Here's how the part is built. I have some questions about the finished solid (model axes, mm). Face numbers are marked on the shaded views. Coordinates: 2 decimals unless noted, no trailing zeros. Loops run counter-clockwise (first coordinate to the right, second up) from the corner with the lowest first, then second, coordinate; pieces in that order, holes last. Notation, with made-up numbers: M 53.25,61 L 97.25,61 A26 cw 97.25,83 Z; hole C -12,73.25 d11. An arc over 180 degrees is marked long. Use CSV: the item, a comma, the result in double quotes. Start each with the question number.
Q1. If we section it at D-D (y = 18): Please give me the cut outline in (x, z).
Q2. If we mould it in two halves opening along X, with no side actions, what happens to the marked faces 1 and 2? For each: +X half, -X half, draft (parallel to the pull), parting line (faces both ways), or undercut.
Q3. If we section it at A-A (x = -1.5): Please give me the cut outline in (y, z), and give its area (3 significant figures).
Q4. For pin 1 Ø11 at (x, y) = (33, 3.5) entering from +Z; pin 2 Ø2.5 at (x, z) = (21.5, 44.5) entering from -Y; pin 3 Ø6 at (x, z) = (18, 24.5) entering from +Y; pin 4 Ø12 at (x, z) = (0, 9) entering from -Y, each with a flat end and sliding along its axis, tell me the tip position at first contact or that it passes through.
Q5. Please list where these lines run through material, in increasing order: probe 1 along Y at (x, z) = (38.5, 33); probe 2 along X at (y, z) = (-96, 35); probe 3 along Y at (x, z) = (4.5, 42.5). Write a range as [from, to].
Q6. If we section it at C-C (z = 45): Please give me the cut outline in (x, y), and give its area (3 significant figures).
Q7. If we section it at B-B (x = 23): State how many separate pieces and enclosed holes the cut face has, and give its area (3 significant figures).
from build123d import *

# Parameters (mm, degrees)
BOSS_EXTRUDE1_DEPTH       = 50
SKETCH2_W                 = 4.7
SKETCH2_H                 = 10
BOSS_EXTRUDE2_DEPTH       = 30
SKETCH3_W                 = 5
SKETCH3_H                 = 50
BOSS_EXTRUDE3_DEPTH       = 120
SKETCH4_W                 = 3
SKETCH4_H                 = 10
BOSS_EXTRUDE4_DEPTH       = 0.25
SKETCH5_W                 = 3
SKETCH5_H                 = 10
BOSS_EXTRUDE5_DEPTH       = 0.25
LPATTERN1_COUNT           = 2
LPATTERN1_PITCH           = 27.6
LPATTERN2_COUNT           = 2
LPATTERN2_PITCH           = 100
LPATTERN2_COPY_1_SKETCH_W = 4.7
LPATTERN2_COPY_1_SKETCH_H = 10
LPATTERN2_COPY_1_DEPTH    = 30
LPATTERN2_COPY_2_SKETCH_W = 3
LPATTERN2_COPY_2_SKETCH_H = 10
LPATTERN2_COPY_2_DEPTH    = 0.25
LPATTERN2_COPY_3_SKETCH_W = 3
LPATTERN2_COPY_3_SKETCH_H = 10
LPATTERN2_COPY_3_DEPTH    = 0.25
CORTE_EXTRUS_O1_DEPTH     = 10
ESBO_O3_W                 = 50
ESBO_O3_H                 = 7.5
RESSALTO_EXTRUS_O2_DEPTH  = 10
ESBO_O4_W                 = 7.5
ESBO_O4_H                 = 45
CORTE_EXTRUS_O2_DEPTH     = 10


with BuildPart() as part:
    # Sketch1 → Boss-Extrude1 (new body)
    with BuildSketch(Plane.XY):
        Polygon((0, 0), (0, 30), (12.8, 30), (12.8, 0), (7.8, 0), (7.8, 10), (6, 10), (6, 0), align=None)
    extrude(amount=BOSS_EXTRUDE1_DEPTH)

    # Sketch2 → Boss-Extrude2 (add)
    with BuildSketch(Plane(origin=(12.8, 0, 0), x_dir=(0, 0, -1), z_dir=(1, 0, 0))):
        with Locations((-45.15, 5)):
            Rectangle(SKETCH2_W, SKETCH2_H)
        with Locations((-32.45, 5)):
            Rectangle(SKETCH2_W, SKETCH2_H)
    boss_extrude2 = extrude(amount=BOSS_EXTRUDE2_DEPTH)

    # Sketch3 → Boss-Extrude3 (add)
    with BuildSketch(Plane.XZ):
        with Locations((10.3, 25)):
            Rectangle(SKETCH3_W, SKETCH3_H)
    extrude(amount=BOSS_EXTRUDE3_DEPTH)

    # Sketch4 → Boss-Extrude4 (add)
    with BuildSketch(Plane(origin=(0, 0, 42.8), x_dir=(-1, 0, 0), z_dir=(0, 0, -1))):
        with Locations((-41.3, 5)):
            Rectangle(SKETCH4_W, SKETCH4_H)
    boss_extrude4 = extrude(amount=BOSS_EXTRUDE4_DEPTH)

    # Sketch5 → Boss-Extrude5 (add)
    with BuildSketch(Plane.XY.offset(34.8)):
        with Locations((41.3, 5)):
            Rectangle(SKETCH5_W, SKETCH5_H)
    boss_extrude5 = extrude(amount=BOSS_EXTRUDE5_DEPTH)

    # LPattern1: Boss-Extrude2, Boss-Extrude4, Boss-Extrude5 ×2
    with Locations(*[(0, 0, -i * LPATTERN1_PITCH) for i in range(1, LPATTERN1_COUNT)]):
        add(boss_extrude2)
        add(boss_extrude4)
        add(boss_extrude5)

    # LPattern2: Boss-Extrude2, Boss-Extrude4, Boss-Extrude5 ×2
    with Locations(*[(0, -i * LPATTERN2_PITCH, 0) for i in range(1, LPATTERN2_COUNT)]):
        add(boss_extrude2)
        add(boss_extrude4)
        add(boss_extrude5)

    # LPattern2 copy 1 sketch → LPattern2 copy 1 (add)
    with BuildSketch(Plane(origin=(12.8, -100, -27.6), x_dir=(0, 0, -1), z_dir=(1, 0, 0))):
        with Locations((-45.15, 5)):
            Rectangle(LPATTERN2_COPY_1_SKETCH_W, LPATTERN2_COPY_1_SKETCH_H)
        with Locations((-32.45, 5)):
            Rectangle(LPATTERN2_COPY_1_SKETCH_W, LPATTERN2_COPY_1_SKETCH_H)
    extrude(amount=LPATTERN2_COPY_1_DEPTH)

    # LPattern2 copy 2 sketch → LPattern2 copy 2 (add)
    with BuildSketch(Plane(origin=(0, -100, 15.2), x_dir=(-1, 0, 0), z_dir=(0, 0, -1))):
        with Locations((-41.3, 5)):
            Rectangle(LPATTERN2_COPY_2_SKETCH_W, LPATTERN2_COPY_2_SKETCH_H)
    extrude(amount=LPATTERN2_COPY_2_DEPTH)

    # LPattern2 copy 3 sketch → LPattern2 copy 3 (add)
    with BuildSketch(Plane(origin=(0, -100, 7.2), x_dir=(1, 0, 0), z_dir=(0, 0, 1))):
        with Locations((41.3, 5)):
            Rectangle(LPATTERN2_COPY_3_SKETCH_W, LPATTERN2_COPY_3_SKETCH_H)
    extrude(amount=LPATTERN2_COPY_3_DEPTH)

    # Esboço2 → Corte-extrusão1 (cut)
    with BuildSketch(Plane.XZ):
        with BuildLine():
            Line((6, 50), (6, 0))
            ThreePointArc((6, 0), (2.708949196, 25), (6, 50))
        make_face()
    extrude(amount=-CORTE_EXTRUS_O1_DEPTH, mode=Mode.SUBTRACT)

    # Esboço3 → Ressalto-extrusão2 (add)
    with BuildSketch(Plane.ZY):
        with Locations((25, 26.25)):
            Rectangle(ESBO_O3_W, ESBO_O3_H)
    extrude(amount=RESSALTO_EXTRUS_O2_DEPTH)

    # Esboço4 → Corte-extrusão2 (cut)
    with BuildSketch(Plane.XZ.offset(-22.5)):
        with Locations((-3.75, 25)):
            Rectangle(ESBO_O4_W, ESBO_O4_H)
    extrude(amount=-CORTE_EXTRUS_O2_DEPTH, mode=Mode.SUBTRACT)


solid = part.part
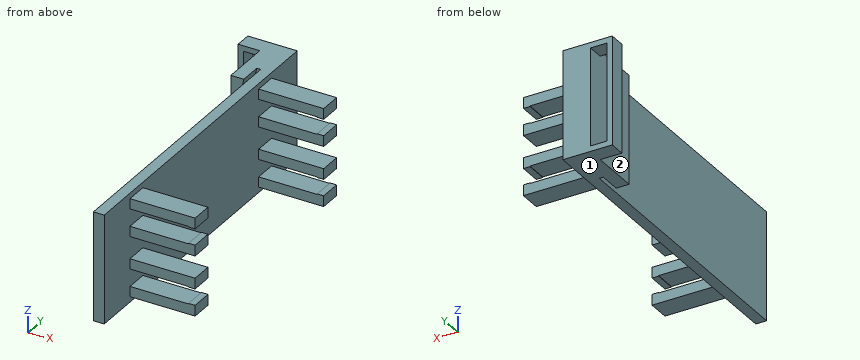
Results below:
1,outline,"M 0,0 L 12.8,0 L 12.8,50 L 0,50 Z"
2,face 1,"draft"
2,face 2,"undercut"
3,outline,"M 22.5,0 L 30,0 L 30,2.5 L 22.5,2.5 Z; M 22.5,47.5 L 30,47.5 L 30,50 L 22.5,50 Z"
3,area,"37.5 mm^2"
4,pin 1,"z = 47.5"
4,pin 2,"y = -100"
4,pin 3,"through"
4,pin 4,"y = 0"
5,probe 1,"[-100, -90], [0, 10]"
5,probe 2,"[7.8, 12.8], [39.8, 42.8]"
5,probe 3,"[10, 30]"
6,outline,"M -10,22.5 L -7.5,22.5 L -7.5,30 L -10,30 Z; M 0,0 L 4.8,0 L 4.8,10 L 7.8,10 L 7.8,-120 L 12.8,-120 L 12.8,-100 L 42.8,-100 L 42.8,-90 L 12.8,-90 L 12.8,0 L 42.8,0 L 42.8,10 L 12.8,10 L 12.8,30 L 0,30 Z"
6,area,"1,570 mm^2"
7,separate pieces,"8"
7,enclosed holes,"0"
7,area,"376 mm^2"
